Could you check a few things on this drawing? It's one solid part, dimensions in mm from its lowest x, y, z. Give positions to 0.01 mm unless a question says otherwise; leave off trailing zeros. Loops run counter-clockwise (first coordinate to the right, second up) from the corner with the lowest first, then second, coordinate; pieces in that order, holes last.
1. Imagine slicing it at B-B (z = 17.05). List the corners of the cut face in (x, y) for me.
2. For P1, Ø1.4, axis at x = 35, y = 3, coming from the -Z side; P2, Ø0.7, axis at y = 7, z = 30.5, coming from the -X side (1 decimal); P3, Ø1, axis at x = 7, y = 2.5, coming from the +Z side (1 decimal), each with a flat end and sliding along its axis, tell me the tip position at first contact or that it passes through.
3. Imagine slicing it at D-D (x = 4). List the corners of the cut face in (y, z) for me.
4. Thinking about a two-plate mould opening in X: for the marked faces 1, 2 and 3, which applies, +X half, -X half, draft (parallel to the pull), parting line (faces both ways), or undercut?
5. Imagine slicing it at A-A (x = 17.05). List the corners of the cut face in (y, z) for me.
6. I need wall thicknesses on line 1 along Z through (x, y) = (17.05, 5.5); line 2 along X through (y, z) = (7.25, 17.05); line 3 along Z through (x, y) = (10, 2.5) (1 decimal). Which ranges of each line are inside material? Lowest first, please.
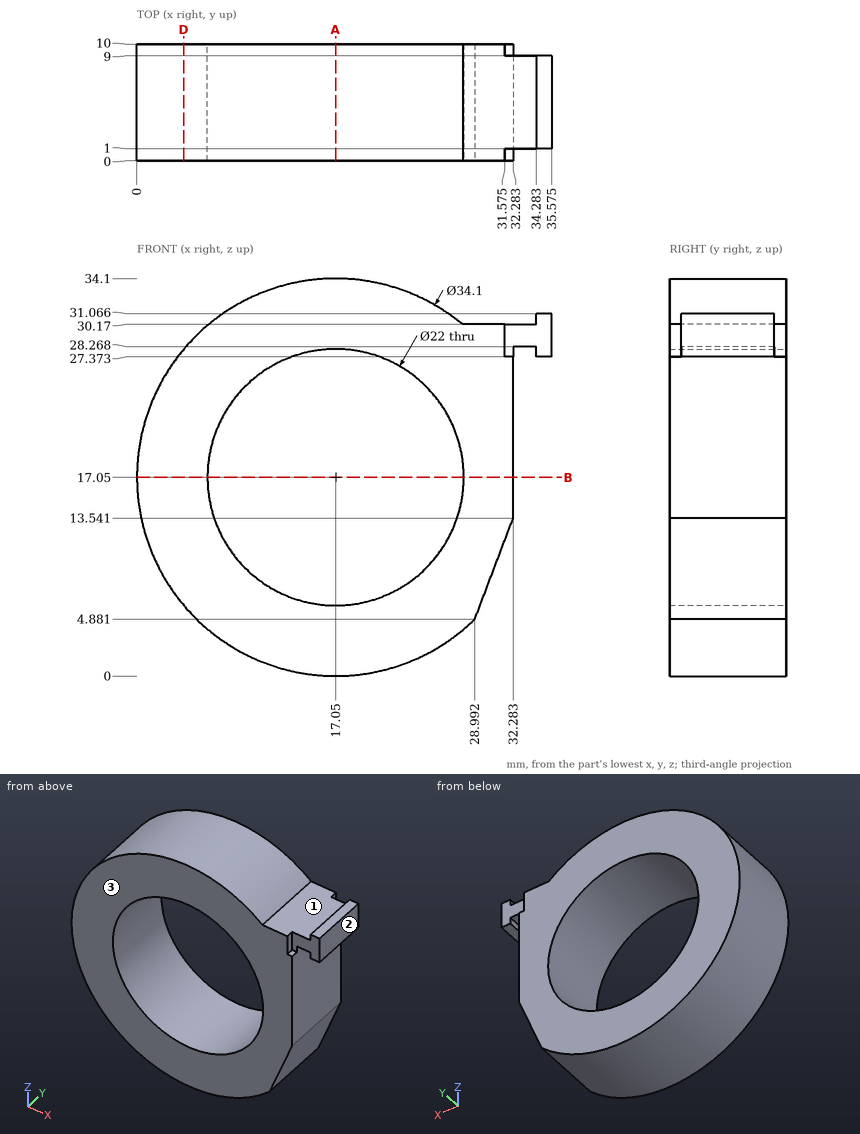
Derived:
1. outline: (0, 0) - (6.05, 0) - (6.05, 10) - (0, 10) - close; (28.05, 0) - (32.28, 0) - (32.28, 10) - (28.05, 10) - close
2. P1: stops at z = 27.37
2. P2: stops at x = 6.1
2. P3: stops at z = 31.2
3. outline: (0, 6.08) - (10, 6.08) - (10, 28.02) - (0, 28.02) - close
4. face 1: undercut
4. face 2: +X half
4. face 3: draft
5. outline: (0, 0) - (10, 0) - (10, 6.05) - (0, 6.05) - close; (0, 28.05) - (10, 28.05) - (10, 34.1) - (0, 34.1) - close
6. line 1: z = 0 to 6.05, 28.05 to 34.1
6. line 2: x = 0 to 6.05, 28.05 to 32.28
6. line 3: z = 1.5 to 8.6, 25.5 to 32.6
